from build123d import *

# Parameters (mm, degrees)
SKETCH_1_R               = 18
SKETCH_1_R_2             = 6.5
EXTRUDE_366_DEPTH        = 4
CUT_EXTRUDE_589_DEPTH    = 3
SKETCH_3_R               = 1.7
CUT_EXTRUDE_770_DEPTH    = 26.632011236
PATTERN_CIRCULAR_1_COUNT = 4
CUT_EXTRUDE_1506_DEPTH   = 3


with BuildPart() as part:
    # Эскиз1 → Extrude 366 (new body)
    with BuildSketch(Plane(origin=(0, 0, 0), x_dir=(1, 0, 0), z_dir=(0, 1, 0))):
        with Locations(Location((0, 0, 0), (0, 0, 270))):
            Circle(SKETCH_1_R)
        with Locations(Location((0, 0, 0), (0, 0, 270))):
            Circle(SKETCH_1_R_2, mode=Mode.SUBTRACT)
    extrude(amount=EXTRUDE_366_DEPTH)

    # Эскиз2 → Cut-Extrude 589 (cut)
    with BuildSketch(Plane(origin=(0, 4, 0), x_dir=(1, 0, 0), z_dir=(0, 1, 0))):
        Polygon((-15.848631561, -2.23e-07), (-14.174315588, -2.900000111), (-10.825684027, -2.899999889), (-9.151368439, 2.23e-07), (-10.825684412, 2.900000111), (-14.174315973, 2.899999889), align=None)
        Polygon((15.848631561, -8.31e-07), (14.174315781, 2.899999169), (10.825684219, 2.899999169), (9.151368439, -8.31e-07), (10.825684219, -2.900000831), (14.174315781, -2.900000831), align=None)
    extrude(amount=-CUT_EXTRUDE_589_DEPTH, mode=Mode.SUBTRACT)

    # Эскиз3 → Cut-Extrude 770 (cut, symmetric)
    with BuildSketch(Plane(origin=(0, 1, 0), x_dir=(1, 0, 0), z_dir=(0, 1, 0))):
        with Locations(Location((12.5, 0, 0), (0, 0, 270))):
            Circle(SKETCH_3_R)
    cut_extrude_770 = extrude(amount=CUT_EXTRUDE_770_DEPTH, both=True, mode=Mode.SUBTRACT)

    # Круговой массив1: Cut-Extrude 770 ×4 about axis
    pattern_circular_1_axis = Axis((0, 0, 0), (0, 1, 0))
    for i in range(1, PATTERN_CIRCULAR_1_COUNT):
        add(cut_extrude_770.rotate(pattern_circular_1_axis, i * 360 / PATTERN_CIRCULAR_1_COUNT), mode=Mode.SUBTRACT)

    # Эскиз5 → Cut-Extrude 1506 (cut)
    with BuildSketch(Plane.XZ):
        Polygon((3.348631561, 12.5), (1.674315781, 15.4), (-1.674315781, 15.4), (-3.348631561, 12.5), (-1.674315781, 9.6), (1.674315781, 9.6), align=None)
        Polygon((-3.348631561, -12.5), (-1.674315781, -15.4), (1.674315781, -15.4), (3.348631561, -12.5), (1.674315781, -9.6), (-1.674315781, -9.6), align=None)
    extrude(amount=-CUT_EXTRUDE_1506_DEPTH, mode=Mode.SUBTRACT)


solid = part.part
Read the model definition and answer for the solid it produces. Units are mm, in the model's axes. A direction names the side the tool comes from. Coordinates: 2 decimals unless noted, no trailing zeros. Order: outer loops, then holes, each group sorted by start corner. A loop starts at its lowest first (then second) coordinate and runs counter-clockwise, first axis right, second up. Notation, with made-up numbers: M 57,63.5 L 88,63.5 A24 cw 88,84.5 Z; hole C -9.75,78.5 d11. An arc over 180 degrees is marked long. Put each result on its own line as item: value. Start each with the question number.
Item 1: Section D-D, the plane x = -5 is taken. Determine the outline of the cut face in (y, z), plus the area to 3 significant figures.
Item 2: Section C-C, the plane x = -12.5 is taken. Determine the outline of the cut face in (y, z).
Item 3: For faces 1 (the face through (-14.186, 0.507, 0.221)), 2 (the face through (2.523, 1.479, 13.93)), 3 (the face through (-9.977, 2.521, -1.43)), determine the directions among +Z, -Z, +X, -X, +Y, -Y from which every point of the face is accessible in a straight line to the end or side of a thin tool.
Item 4: Section A-A, the plane x = 0 is taken. Determine the outline of the cut face in (y, z).
Item 5: The mould has two halves that part along Z. Classify faces 4 (the face through (0, 1, -9.6)), 5 (the face through (-8, 4, 0)): +Z half, -Z half, draft (parallel to the pull), parting line (faces both ways), or undercut.
Item 6: Given pin 1 Ø1 at (x, y) = (13.5, 0.5) entering from +Z; pin 2 Ø4.5 at (x, z) = (12, 0) entering from +Y; pin 3 Ø11.5 at (x, z) = (0, 0) entering from +Y; pin 4 Ø1.5 at (x, y) = (8.5, 3.5) entering from +Z, each flat-ended and moving along its own axis, determine where each tip first touches the part or whether it passes through.
Item 7: Consider probe 1 along X at (y, z) = (0.7, 0); probe 2 along X at (y, z) = (0.4, 2); probe 3 along Z at (x, y) = (-10, 1.4). Determine where each line is inside the solid, lowest interval first. Write a range as [from, to].
Item 8: Section B-B, the plane z = 4.5 is taken. Determine the outline of the cut face in (x, y), plus the area to 3 significant figures.
Computed:
1. outline: M 0,-17.29 L 4,-17.29 L 4,-4.15 L 0,-4.15 Z; M 0,4.15 L 4,4.15 L 4,17.29 L 0,17.29 Z
1. area: 105 mm2
2. outline: M 0,-12.95 L 4,-12.95 L 4,-2.9 L 1,-2.9 L 1,-1.7 L 0,-1.7 Z; M 0,1.7 L 1,1.7 L 1,2.9 L 4,2.9 L 4,12.95 L 0,12.95 Z
3. face 1: +Y, -Y
3. face 2: -Y
3. face 3: +Y
4. outline: M 0,-18 L 4,-18 L 4,-14.2 L 3,-14.2 L 3,-15.4 L 0,-15.4 Z; M 0,-9.6 L 3,-9.6 L 3,-10.8 L 4,-10.8 L 4,-6.5 L 0,-6.5 Z; M 0,6.5 L 4,6.5 L 4,10.8 L 3,10.8 L 3,9.6 L 0,9.6 Z; M 0,15.4 L 3,15.4 L 3,14.2 L 4,14.2 L 4,18 L 0,18 Z
5. face 4: undercut
5. face 5: draft
6. pin 1: stops at z = 12.45
6. pin 2: stops at y = 1
6. pin 3: passes through
6. pin 4: stops at z = 16.25
7. probe 1: x = [-18, -14.2], [-10.8, -6.5], [6.5, 10.8], [14.2, 18]
7. probe 2: x = [-17.89, -6.18], [6.18, 17.89]
7. probe 3: z = [-14.97, -1.47], [1.47, 14.97]
8. outline: M -17.43,0 L -4.69,0 L -4.69,4 L -17.43,4 Z; M 4.69,0 L 17.43,0 L 17.43,4 L 4.69,4 Z
8. area: 102 mm2
